CAD build for the part. Positions are in the model's coordinates, mm. A direction names the side the tool comes from. Round coordinates to 2 decimals unless told otherwise and drop trailing zeros. Write each loop counter-clockwise with the first axis right and the second up, starting at its lowest first coordinate (ties: lowest second). Pieces come first, ordered by that corner, then holes. Notation, with made-up numbers: (24, -29.5) - (34, -29.5) arc R23 ccw to (34, 6.5) - close; hole circle Ø8 at (-22, -4). An arc over 180 degrees is marked (long way). Use one line per item in the form item = value. Start each with the question number.
Item 1: Band-saw the part on A-A, the plane y = 79. List the corners of the cut face in (x, z).
Item 2: Band-saw the part on B-B, the plane z = -5. List the corners of the cut face in (x, y), and give its area (3 significant figures).
Item 3: Tool access for faces 1 (the flat face through (114.719, -11.475, -3.506)), 2 (the cylindrical face through (29, -8, -4)): list every direction of +Z, -Z, +X, -X, +Y, -Y with a clear straight run to the whole face (end or side of a thin tool).
Item 4: Pin check, flat tips, straight feed: pin 1 (2 mm diameter, centred on y = -4, z = -4.5, fed in from +X); pin 2 (8 mm diameter, centred on x = 23, y = 28, fed in from -Z); pin 3 (1 mm diameter, centred on y = -4.5, z = -5, fed in from -X). Stop position of each tip, or through.
Item 5: Pull direction X, two halves, no side cores. Call faces 3 (the cylindrical face through (-108.98, 28.65, -3.61)), 4 (the cylindrical face through (-151.098, -14.297, -3.606)), 5 (the cylindrical face through (66.185, -19.556, -3.606)), 6 (the flat face through (-42, -20, -4)): +X half, -X half, draft (parallel to the pull), parting line (faces both ways), or undercut.
Item 6: Drill centre lines: L1, parallel to Y at x = 0.5, z = -3.25; L2, parallel to Y at x = 34, z = -2.5; L3, parallel to Y at x = -85, z = -5.25. Where is each one in solid material? Low to high.
from build123d import *

# Parameters (mm, degrees)
SKETCH1_W               = 314.224
SKETCH1_H               = 280
BOSS_EXTRUDE1_DEPTH     = 7.112
CUT_EXTRUDE1_DEPTH      = 304.866353991
CUT_EXTRUDE1_DEPTH_BACK = 304.866353991
CUT_EXTRUDE2_DEPTH      = 304.866353991
CUT_EXTRUDE3_DEPTH      = 304.866353991
FILLET1_R               = 120
FILLET2_R               = 20
FILLET3_R               = 4
CUT_EXTRUDE4_DEPTH      = 304.866353991


with BuildPart() as part:
    # Sketch1 → Boss-Extrude1 (new body)
    with BuildSketch(Plane(origin=(0, 0, 0), x_dir=(1, 0, 0), z_dir=(0, 0, -1))):
        with Locations((0, -120)):
            Rectangle(SKETCH1_W, SKETCH1_H)
    extrude(amount=BOSS_EXTRUDE1_DEPTH)

    # Sketch2 → Cut-Extrude1 (cut, two sides: drawn at the far end of the back side and taken through both)
    with BuildSketch(Plane.XY.offset(-CUT_EXTRUDE1_DEPTH_BACK)):
        with BuildLine():
            Line((-101.985505074, 143.817457954), (98.803851758, 143.817457954))
            ThreePointArc((98.803851758, 143.817457954), (105.87491957, 140.888525766), (108.803851758, 133.817457954))
            Line((108.803851758, 133.817457954), (108.803851758, 35.797968831))
            ThreePointArc((108.803851758, 35.797968831), (105.87491957, 28.726901019), (98.803851758, 25.797968831))
            Line((98.803851758, 25.797968831), (-101.985505074, 25.797968831))
            ThreePointArc((-101.985505074, 25.797968831), (-109.056572886, 28.726901019), (-111.985505074, 35.797968831))
            Line((-111.985505074, 35.797968831), (-111.985505074, 133.817457954))
            ThreePointArc((-111.985505074, 133.817457954), (-109.056572886, 140.888525766), (-101.985505074, 143.817457954))
        make_face()
    extrude(amount=CUT_EXTRUDE1_DEPTH + CUT_EXTRUDE1_DEPTH_BACK, mode=Mode.SUBTRACT)

    # Sketch3 → Cut-Extrude2 (cut, through all)
    with BuildSketch(Plane.XY):
        with BuildLine():
            Line((-12, -8), (12, -8))
            ThreePointArc((12, -8), (14.121320344, -7.121320344), (15, -5))
            Line((15, -5), (15, -3))
            ThreePointArc((15, -3), (14.121320344, -0.878679656), (12, 0))
            Line((12, 0), (-12, 0))
            ThreePointArc((-12, 0), (-14.121320344, -0.878679656), (-15, -3))
            Line((-15, -3), (-15, -5))
            ThreePointArc((-15, -5), (-14.121320344, -7.121320344), (-12, -8))
        make_face()
    extrude(amount=-CUT_EXTRUDE2_DEPTH, mode=Mode.SUBTRACT)

    # Sketch4 → Cut-Extrude3 (cut, through all)
    with BuildSketch(Plane.XY):
        Polygon((66.371490886, -20), (157.112, -4), (157.112, -20), align=None)
    extrude(amount=-CUT_EXTRUDE3_DEPTH, mode=Mode.SUBTRACT)

    # Fillet1
    fillet1_edges = [part.edges().sort_by_distance(p)[0] for p in [
        (66.371490886, -20, -3.556),
    ]]
    fillet(fillet1_edges, radius=FILLET1_R)

    # Fillet2
    fillet2_edges = [part.edges().sort_by_distance(p)[0] for p in [
        (-157.112, -20, -3.556),
    ]]
    fillet(fillet2_edges, radius=FILLET2_R)

    # Fillet3
    fillet3_edges = [part.edges().sort_by_distance(p)[0] for p in [
        (157.112, -4, -3.556),
    ]]
    fillet(fillet3_edges, radius=FILLET3_R)

    # Sketch5 → Cut-Extrude4 (cut, through all)
    with BuildSketch(Plane.XY):
        with BuildLine():
            Line((35, -2), (65, -2))
            ThreePointArc((65, -2), (71, -8), (65, -14))
            Line((65, -14), (35, -14))
            ThreePointArc((35, -14), (29, -8), (35, -2))
        make_face()
    extrude(amount=-CUT_EXTRUDE4_DEPTH, mode=Mode.SUBTRACT)


solid = part.part
Determined:
q1.outline = (-157.11, -7.11) - (-111.99, -7.11) - (-111.99, 0) - (-157.11, 0) - close; (108.8, -7.11) - (157.11, -7.11) - (157.11, 0) - (108.8, 0) - close
q2.outline = (-157.11, 0) arc R20 ccw to (-137.11, -20) - (55.87, -20) arc R120 ccw to (76.71, -18.18) - (153.81, -4.58) arc R4 ccw to (157.11, -0.64) - (157.11, 260) - (-157.11, 260) - close; hole (-111.99, 35.8) arc R10 ccw to (-101.99, 25.8) - (98.8, 25.8) arc R10 ccw to (108.8, 35.8) - (108.8, 133.82) arc R10 ccw to (98.8, 143.82) - (-101.99, 143.82) arc R10 ccw to (-111.99, 133.82) - close; hole (-15, -5) arc R3 ccw to (-12, -8) - (12, -8) arc R3 ccw to (15, -5) - (15, -3) arc R3 ccw to (12, 0) - (-12, 0) arc R3 ccw to (-15, -3) - close; hole (35, -14) - (65, -14) arc R6 ccw to (65, -2) - (35, -2) arc R6 ccw to start
q2.area = 60,500 mm²
q3.face_1 = +Z, -Z, +X, -Y
q3.face_2 = +Z, -Z
q4.pin_1 = 156.34
q4.pin_2 = -7.11
q4.pin_3 = -156.71
q5.face_3 = undercut
q5.face_4 = -X half
q5.face_5 = +X half
q5.face_6 = draft
q6.L1 = -20 to -8, 0 to 25.8, 143.82 to 260
q6.L2 = -20 to -13.92, -2.08 to 25.8, 143.82 to 260
q6.L3 = -20 to 25.8, 143.82 to 260
